from build123d import *

# Parameters (mm, degrees)
FILLET1_R = 0.4445


with BuildPart() as part:
    # Sweep1: sweep along a path in Sketch1
    with BuildLine(Plane(origin=(0, 0, 0), x_dir=(1, 0, 0), z_dir=(0, 1, 0))) as sweep1_path:
        ThreePointArc((5.588, 0), (7.231440893, 8.262135305), (11.911564594, 15.266435406))
    # Sketch2 → Sweep1 (sweep)
    with BuildSketch(Plane.XY):
        with BuildLine():
            ThreePointArc((11.326, 0), (7.714353036, 5.329471528), (1.425941872, 3.949926093))
            ThreePointArc((1.425941872, 3.949926093), (14.732551814, 0), (1.425941872, -3.949926093))
            ThreePointArc((1.425941872, -3.949926093), (7.714353036, -5.329471528), (11.326, 0))
        make_face()
    sweep(path=sweep1_path.line)

    # Fillet1
    fillet1_edges = [part.edges().sort_by_distance(p)[0] for p in [
        (3.386200576, 3.949926093, -9.854885995),
        (3.386200576, -3.949926093, -9.854885995),
    ]]
    fillet(fillet1_edges, radius=FILLET1_R)


solid = part.part
Here's how the part is built. I have some questions about the finished solid (model axes, mm). Coordinates: 2 decimals unless noted, no trailing zeros. Write each loop counter-clockwise with the first axis right and the second up, starting at its lowest first coordinate (ties: lowest second). Pieces come first, ordered by that corner, then holes.
1) I'm going to push flat-ended pins straight in: pin 1 (5 mm diameter, centred on x = 5.5, z = -2.5, fed in from -Y); pin 2 (3 mm diameter, centred on y = 5.5, z = -8.5, fed in from +X); pin 3 (1 mm diameter, centred on y = -4, z = -9, fed in from -X); pin 4 (2 mm diameter, centred on x = 9.5, z = -5.5, fed in from +Y). Where does each tip first touch, or does it pass through?
Filled in:
pin 1: stops at y = -7.24
pin 2: stops at x = 17
pin 3: stops at x = 11.5
pin 4: stops at y = 7.24
2) If we section it at B-B (y = -0.25): List the corners of the cut face in (x, z) for me, plus the area to 3 significant figures.
Filled in:
outline: (11.32, 0) arc R15.86 ccw to (15.97, -11.21) - (18.37, -8.8) arc R12.45 cw to (14.73, 0) - close
area: 37.9 mm2
3) If I drill on line 1 (Y direction, x = 10, z = -9.75); line 2 (Y direction, x = 13, z = -9); line 3 (X direction, y = -3.25, z = -3), over which ranges is the centre line in solid material (lowest first)?
Filled in:
line 1: y = -7.24 to -5.44, 5.44 to 7.24
line 2: y = -6.64 to -3.15, 3.15 to 6.64
line 3: x = 10.59 to 14.31
4) If we section it at A-A (y = 2): List the corners of the cut face in (x, z) for me.
Filled in:
outline: (10.97, 0) arc R16.21 ccw to (15.71, -11.46) - (18.18, -9) arc R12.73 cw to (14.45, 0) - close
